Autodesk Fusion 360 part; units mm, degrees
sketch "bottom" plane through (0, 0, 0) normal (0, 0, 1) x (1, 0, 0)
  line L0 (44, -44) -> (-44, -44)
  line L1 (-44, -44) -> (-44, 44)
  line L2 (-44, 44) -> (44, 44)
  line L3 (44, 44) -> (44, -44)
  line L4 (44, -44) -> (-44, 44) construction
  line L5 (-44, -44) -> (44, 44) construction
  dimension "d1" = 88
  dimension "d2" = 88
extrude "Extrude1" add sketch "bottom" along normal blind 10
sketch "Sketch2" plane through (0, 0, 10) normal (0, 0, 1) x (-1, 0, 0)
  line L0 (-44, -44) -> (44, -44)
  line L1 (44, -44) -> (44, 44)
  line L2 (44, 44) -> (-44, 44)
  line L3 (-44, 44) -> (-44, -44)
  line L4 (-44, 0) -> (-25, 0)
  circle A0 centre (-25, 0) radius 19
chamfer "Chamfer1" distance 36 angle 45 2 edges at (44, -44, 5) (44, 44, 5)
fillet "Fillet1" radius 19 2 edges at (44, -8, 5) (44, 8, 5)
sketch "Sketch3" plane through (0, 0, 10) normal (0, 0, 1) x (-1, 0, 0)
  line L0 (44, 44) -> (31, 44)
  line L1 (31, 44) -> (31, -44)
  line L2 (31, -44) -> (44, -44)
  line L3 (44, -44) -> (44, 44)
extrude "Extrude2" add sketch "Sketch3" along normal blind 40
sketch "Sketch4" plane through (0, 0, 10) normal (0, 0, 1) x (-1, 0, 0)
  line L0 (31, -44) -> (31, 44)
  line L1 (31, 44) -> (-8, 44)
  line L2 (-8, 44) -> (-38.435, 13.565)
  arc A0 (-38.435, 13.565) -> (-44, 0.1299) centre (-25, 0.1299) ccw
  line L3 (-44, 0.1299) -> (-44, -0.1299)
  arc A1 (-44, -0.1299) -> (-38.435, -13.565) centre (-25, -0.1299) ccw
  line L4 (-38.435, -13.565) -> (-8, -44)
  line L5 (-8, -44) -> (31, -44)
  line L6 (28, -22) -> (31, -22)
  line L7 (31, -22) -> (31, 22)
  line L8 (31, 22) -> (28, 22)
  line L9 (28, 22) -> (28, -22)
  dimension "d12" = 3
extrude "Extrude3" add sketch "Sketch4" along normal blind 40 contours L0 L6 L7 L8 L9
fillet "Fillet2" radius 3 1 edges at (-31, -22, 30)
fillet "Fillet3" radius 3 1 edges at (-31, 22, 30)
sketch "Sketch6" plane through (0, 0, 0) normal (0, 1, 0) x (1, 0, 0)
  line L0 (-28, -50) -> (-24, -50)
  line L1 (-24, -50) -> (-24, -10)
  line L2 (-24, -10) -> (-28, -10)
  line L3 (-28, -10) -> (-28, -50)
  dimension "d19" = 40
extrude "Extrude4" add sketch "Sketch6" along normal mid plane 10
sketch "triangle" plane through (0, -5, 0) normal (0, -1, 0) x (1, 0, 0)
  line L0 (-28, 50) -> (-28, 10)
  line L1 (-28, 10) -> (-24, 10)
  line L2 (-24, 10) -> (-24, 50)
  line L3 (-24, 50) -> (-28, 50)
  line L4 (-24, 50) -> (-24, 10)
  line L5 (-24, 10) -> (25, 10)
  line L6 (25, 10) -> (-24, 50)
  line L7 (44, 10) -> (25, 10)
  dimension "d26" = 19
  dimension "d28" = 49
extrude "Extrude5" add sketch "triangle" against normal blind 10 contours L2 L4 L5 L6
sketch "the back" plane through (-44, 0, 0) normal (-1, 0, 0) x (0, -1, 0)
  line L0 (-44, 0) -> (44, 0)
  line L1 (44, 0) -> (44, 50)
  line L2 (44, 50) -> (-44, 50)
  line L3 (-44, 50) -> (-44, 0)
  line L4 (-19, 50) -> (19, 50)
  line L5 (19, 50) -> (19, 0)
  line L6 (19, 0) -> (-19, 0)
  line L7 (-19, 0) -> (-19, 50)
extrude "Extrude6" add sketch "the back" along normal blind 19 contours L0 L2 L4 L5 L6 L7
fillet "Fillet4" radius 6 1 edges at (-44, -19, 25)
fillet "Fillet5" radius 6 1 edges at (-44, 19, 25)
fillet "Fillet6" radius 19 2 edges at (-63, 19, 25) (-63, -19, 25)
sketch "wall circle" plane through (0, 0, 50) normal (0, 0, 1) x (-1, 0, 0)
  arc A0 (63, 0.7307) -> (48.56, 19.1754) centre (44, 0.7307) ccw
  arc A1 (44, 25) -> (48.56, 19.1754) centre (50, 25) ccw
  line L0 (44, 25) -> (44, 44)
  line L1 (44, 44) -> (31, 44)
  line L2 (31, 44) -> (31, 25)
  arc A2 (28, 22) -> (31, 25) centre (28, 25) ccw
  line L3 (28, 22) -> (28, 5)
  line L4 (28, 5) -> (24, 5)
  line L5 (24, 5) -> (24, -5)
  line L6 (24, -5) -> (28, -5)
  line L7 (28, -5) -> (28, -22)
  arc A3 (31, -25) -> (28, -22) centre (28, -25) ccw
  line L8 (31, -25) -> (31, -44)
  line L9 (31, -44) -> (44, -44)
  line L10 (44, -44) -> (44, -25)
  arc A4 (48.56, -19.1754) -> (44, -25) centre (50, -25) ccw
  arc A5 (48.56, -19.1754) -> (63, -0.7307) centre (44, -0.7307) ccw
  line L11 (63, -0.7307) -> (63, 0.7307)
  circle A6 centre (46.3334, -0.7307) radius 9.5
  dimension "d37" = 19
extrude "Extrude7" cut sketch "wall circle" against normal blind 50 contours A6
sketch "bottom circles" plane through (0, 0, 10) normal (0, 0, 1) x (-1, 0, 0)
  line L0 (-25, 5) -> (28, 5)
  line L1 (28, 5) -> (28, 22)
  arc A0 (28, 22) -> (31, 25) centre (28, 25) ccw
  line L2 (31, 25) -> (31, 44)
  line L3 (31, 44) -> (-8, 44)
  line L4 (-8, 44) -> (-38.435, 13.565)
  arc A1 (-38.435, 13.565) -> (-44, 0.1299) centre (-25, 0.1299) ccw
  line L5 (-44, 0.1299) -> (-44, -0.1299)
  arc A2 (-44, -0.1299) -> (-38.435, -13.565) centre (-25, -0.1299) ccw
  line L6 (-38.435, -13.565) -> (-8, -44)
  line L7 (-8, -44) -> (31, -44)
  line L8 (31, -44) -> (31, -25)
  arc A3 (31, -25) -> (28, -22) centre (28, -25) ccw
  line L9 (28, -22) -> (28, -5)
  line L10 (28, -5) -> (-25, -5)
  line L11 (-25, -5) -> (-25, 5)
  circle A4 centre (0.1969, 25) radius 5
  circle A5 centre (0, -25) radius 5
  dimension "d43" = 10
  dimension "d44" = 10
extrude "Extrude8" cut sketch "bottom circles" against normal blind 10 contours A4 | A5
Here's how the part is built. I have some questions about the finished solid (model axes, mm). A direction names the side the tool comes from. Coordinates: 2 decimals unless noted, no trailing zeros. Order: outer loops, then holes, each group sorted by start corner. A loop starts at its lowest first (then second) coordinate and runs counter-clockwise, first axis right, second up. Notation, with made-up numbers: M -2.75,19 L 35.25,19 A16 cw 35.25,32 Z; hole C 66.5,-35.75 d11. An arc over 180 degrees is marked long. Answer as CSV lines item,"result". Start each with the question number.
1. On a 3-axis mill with a long thin cutter (end or side, diameter ignored), from which of +Z, -Z, +X, -X, +Y, -Y can I reach the whole of each face in a straight line? I mean faces 4 (the flat face through (-44, 35, 25)), 5 (the flat face through (-44, -34, 25)), 6 (the flat face through (-31, 34, 30)), 7 (the flat face through (-28, -14, 30)), 8 (the cylindrical face through (42.513, -7.497, 5.07)). Say none if no direction works.
2. I want a section at B-B, the plane z = 5.5. Count the separate pieces of the cut face and the enclosed holes in it, and give its area (3 significant figures).
3. We'd pull the mould along Y, two halves only. Please class faces 1 (the cylindrical face through (1.08, 29.88, 5.07)), 2 (the flat face through (23, 29, 5)), 3 (the flat face through (-2, 10, 10)): released by +Y, released by -Y, zero draft, split by the parting line, or undercut.
4. For pin 1 (5 mm diameter, centred on x = -9, y = 14, fed in from +Z); pin 2 (9.5 mm diameter, centred on y = 30.5, z = 24.5, fed in from +X); pin 3 (12 mm diameter, centred on y = -28, z = 32, fed in from -X); pin 4 (12 mm diameter, centred on x = -46.5, y = -17, fed in from -Z), each with a flat end and sliding along its axis, tell me the tip position at first contact or that it passes through.
5. I want a section at A-A, the plane x = 0. Write out the boundary of the cut face in (y, z).
6. I need wall thicknesses on line 1 (Y direction, x = 0, z = 3); line 2 (Y direction, x = 2, z = 4); line 3 (Z direction, x = -16, y = -40). Which ranges of each line are inside material? Lowest first, please. Write a range as [from, to].
Recorded:
1,face 4,"+Z, -Z, -X, +Y"
1,face 5,"+Z, -Z, -X, -Y"
1,face 6,"+Z, +X, +Y"
1,face 7,"+Z, +X, -Y"
1,face 8,"+Z, -Z, +X, -Y"
2,separate pieces,"1"
2,enclosed holes,"3"
2,area,"6,600 mm2"
3,face 1,"undercut"
3,face 2,"released by +Y"
3,face 3,"zero draft"
4,pin 1,"stops at z = 10"
4,pin 2,"stops at x = -31"
4,pin 3,"stops at x = -44.8"
4,pin 4,"stops at z = 0"
5,outline,"M -44,0 L -30,0 L -30,10 L -44,10 Z; M -20,0 L 20,0 L 20,10 L 5,10 L 5,30.41 L -5,30.41 L -5,10 L -20,10 Z; M 30,0 L 44,0 L 44,10 L 30,10 Z"
6,line 1,"y = [-44, -30], [-20, 20], [30, 44]"
6,line 2,"y = [-44, -29.49], [-20.51, 20.42], [29.58, 44]"
6,line 3,"z = [0, 10]"
